from build123d import *

# Parameters (mm, degrees)
SKETCH_1_R           = 50
SKETCH_1_R_2         = 42.5
EXTRUDE_1_DEPTH      = 50
SKETCH_1_2_R         = 50
SKETCH_1_2_R_2       = 42.5
EXTRUDE_2_DEPTH      = 100
EXTRUDE_3_REACH      = 189.083
EXTRUDE_3_END_RADIUS = 50
SKETCH_2_R           = 50
SKETCH_2_R_2         = 42.5
SKETCH_3_R           = 42.5
CUT_EXTRUDE_1_DEPTH  = 200
SKETCH_3_2_R         = 42.5
CUT_EXTRUDE_2_DEPTH  = 100


with BuildPart() as part:
    # 草图1 → 凸台-拉伸1 (new, symmetric)
    with BuildSketch(Plane(origin=(0, 0, 0), x_dir=(0, 0, -1), z_dir=(1, 0, 0))):
        Circle(SKETCH_1_R)
        Circle(SKETCH_1_R_2, mode=Mode.SUBTRACT)
    extrude(amount=EXTRUDE_1_DEPTH, both=True)

    # 草图1<2> → 凸台-拉伸2 (add, symmetric)
    with BuildSketch(Plane(origin=(0, 0, 0), x_dir=(0, 0, -1), z_dir=(1, 0, 0))):
        Circle(SKETCH_1_2_R)
        Circle(SKETCH_1_2_R_2, mode=Mode.SUBTRACT)
    extrude(amount=EXTRUDE_2_DEPTH, both=True)

    # 凸台-拉伸3: up to this cylinder (the profile starts outside it)
    extrude_3_end = Plane(origin=(0, 0, 0), z_dir=(-1, 0, 0)) * Cylinder(EXTRUDE_3_END_RADIUS, 479.166, mode=Mode.PRIVATE)
    # 草图2 → 凸台-拉伸3 (add, up to the surface)
    with BuildSketch(Plane(origin=(0, 100, 0), x_dir=(1, 0, 0), z_dir=(0, 1, 0)), mode=Mode.PRIVATE) as extrude_3_sk1:
        with Locations(Location((0, 0, 0), (0, 0, 270))):
            Circle(SKETCH_2_R)
        with Locations(Location((0, 0, 0), (0, 0, 270))):
            Circle(SKETCH_2_R_2, mode=Mode.SUBTRACT)
    extrude_3_tool1 = extrude(extrude_3_sk1.sketch, amount=-EXTRUDE_3_REACH, mode=Mode.PRIVATE) - extrude_3_end
    add(extrude_3_tool1.solids().sort_by_distance((0, 100, -48.585786))[0])

    # 草图3 → 切除-拉伸1 (cut)
    with BuildSketch(Plane(origin=(0, 0, 0), x_dir=(1, 0, 0), z_dir=(0, 1, 0))):
        with Locations(Location((0, 0, 0), (0, 0, 270))):
            Circle(SKETCH_3_R)
    extrude(amount=-CUT_EXTRUDE_1_DEPTH, mode=Mode.SUBTRACT)

    # 草图3<2> → 切除-拉伸2 (cut, symmetric)
    with BuildSketch(Plane(origin=(0, 0, 0), x_dir=(1, 0, 0), z_dir=(0, 1, 0))):
        with Locations(Location((0, 0, 0), (0, 0, 270))):
            Circle(SKETCH_3_2_R)
    extrude(amount=CUT_EXTRUDE_2_DEPTH, both=True, mode=Mode.SUBTRACT)


solid = part.part
Can you work these out from the model? Positions are in its coordinate system, mm. A direction names the side the tool comes from. Coordinates: 2 decimals unless noted, no trailing zeros. Loops run counter-clockwise (first coordinate to the right, second up) from the corner with the lowest first, then second, coordinate; pieces in that order, holes last. Notation, with made-up numbers: (67, -11.5) - (84, -11.5) arc R26 ccw to (84, 18.5) - close; hole circle Ø4 at (58.5, 28.25). An arc over 180 degrees is marked (long way). Put each result on its own line as item: value. Start each with the question number.
Item 1: Which directions (+Z, -Z, +X, -X, +Y, -Y) give clear straight access to the entire face, cutting with the end or side of a thin tool? Please do faces 1 (the face through (-100, -37, 22)), 2 (the face through (33.792, 61.811, -36.852)).
Item 2: Suppose I cut it at B-B (y = 10). Please give me the cut outline in (x, z), and give its area (3 significant figures).
Item 3: Suppose I cut it at A-A (z = 0). Please give me the cut outline in (x, y).
Item 4: Suppose I cut it at C-C (x = -24.5). Please give me the cut outline in (y, z).
Item 5: Suppose I cut it at D-D (x = 74). Please give me the cut outline in (y, z), and give its area (3 significant figures).
Item 6: If I drill on line 1 along Z through (x, y) = (32.5, 0); line 2 along Y through (x, z) = (49, 0); line 3 along Z through (x, y) = (-8, 74.5), over which ranges is the centre line in solid material (lowest first)?
Item 7: For pin 1 (2 mm diameter, centred on x = 52.5, z = 12.5, fed in from +Y); pin 2 (8 mm diameter, centred on x = 46.5, z = -20, fed in from -Y); pin 3 (4 mm diameter, centred on x = -55, z = -23, fed in from -Y), each with a flat end and sliding along its axis, tell me the tip position at first contact or that it passes through.
Item 8: If we mould it in two halves opening along Y, with no side actions, what happens to faces 3 (the face through (-61.811, -37.705, -19.611)), 4 (the face through (1.4, -19.15, -46.187)), 5 (the face through (100, -37, 22))? For each: +Y half, -Y half, draft (parallel to the pull), parting line (faces both ways), or undercut.
Here are the results:
1. face 1: +Z, -Z, -X, +Y, -Y
1. face 2: +Y
2. outline: (-100, -48.99) - (-10, -48.99) arc R50 ccw to (10, -48.99) - (100, -48.99) - (100, -41.31) - (10, -41.31) arc R42.5 cw to (-10, -41.31) - (-100, -41.31) - close; (-100, 41.31) - (-10, 41.31) arc R42.5 cw to (10, 41.31) - (100, 41.31) - (100, 48.99) - (10, 48.99) arc R50 ccw to (-10, 48.99) - (-100, 48.99) - close
2. area: 3,070 mm²
3. outline: (-100, -50) - (-42.5, -50) - (-42.5, -42.5) - (-100, -42.5) - close; (-100, 42.5) - (-42.5, 42.5) - (-42.5, 100) - (-50, 100) - (-50, 50) - (-100, 50) - close; (42.5, -50) - (100, -50) - (100, -42.5) - (42.5, -42.5) - close; (42.5, 42.5) - (100, 42.5) - (100, 50) - (50, 50) - (50, 100) - (42.5, 100) - close
4. outline: (-35.97, -34.73) arc R50 ccw to (24.5, -43.59) - (100, -43.59) - (100, -34.73) - (24.5, -34.73) arc R42.5 cw to (-24.5, -34.73) - close; (-35.97, 34.73) - (-24.5, 34.73) arc R42.5 cw to (24.5, 34.73) - (100, 34.73) - (100, 43.59) - (24.5, 43.59) arc R50 ccw to start
5. outline: circle Ø100 at (0, 0); hole circle Ø85 at (0, 0)
5. area: 2,180 mm²
6. line 1: -50 to -42.5, 42.5 to 50
6. line 2: -50 to -42.5, 42.5 to 100
6. line 3: -49.36 to -41.74, 41.74 to 49.36
7. pin 1: y = 48.66
7. pin 2: y = -47.37
7. pin 3: y = -45.38
8. face 3: undercut
8. face 4: parting line
8. face 5: draft
